Part model, mm, in its own coordinate system. A direction names the side the tool comes from. Coordinates: 2 decimals unless noted, no trailing zeros. Loops run counter-clockwise (first coordinate to the right, second up) from the corner with the lowest first, then second, coordinate; pieces in that order, holes last. Notation, with made-up numbers: M -23,6 L 16,6 A18 ccw 16,29 Z; hole C 28,46.25 d7. An arc over 180 degrees is marked long. Answer as CSV lines item,"result". Start each with the question number.
Autodesk Inventor part; units mm, degrees
ref_plane "Work Plane3" through (64.8592, 82.2824, 5) normal (0.5, 0, -0.866) x (0, 1, 0)
ref_plane "YZ Plane" through (0, 0, 0) normal (1, 0, 0) x (0, 1, 0)
ref_plane "XZ Plane" through (0, 0, 0) normal (0, 1, 0) x (-1, 0, 0)
sketch "Sketch1" plane through (0, 0, 0) normal (0, 0, 1) x (1, 0, 0)
  line L0 (0, 0) -> (55, 95.2628)
  line L1 (0, 0) -> (8.6603, 0)
  line L2 (64.8592, 0) -> (64.8592, 115) construction
  line L3 (64.8592, 0) -> (179.8592, 0) construction
  line L4 (56.1603, 82.2724) -> (65.4694, 82.2724) construction
  line L5 (79.2606, 82.2724) -> (79.2606, 95.2628)
  line L6 (55, 95.2628) -> (79.2606, 95.2628)
  line L7 (64.8592, 82.2724) -> (64.8592, 82.2824) construction
  line L8 (64.8592, 82.2824) -> (64.865, 82.2724)
  line L9 (64.8592, 82.2824) -> (64.8707, 82.2824) construction
  line L10 (64.8592, 82.2824) -> (64.8534, 82.2724)
  line L11 (64.8592, 82.2824) -> (64.8707, 82.2824) construction
  line L12 (64.865, 82.2724) -> (79.2606, 82.2724)
  line L13 (56.1603, 82.2724) -> (64.8534, 82.2724)
  line L14 (8.6603, 0) -> (53.6603, 0) construction
  line L15 (53.6603, 0) -> (32.0862, 40.5749)
  line L16 (53.6603, 0) -> (99.6142, 0) construction
  line L17 (36.5081, 48.2339) -> (62.1545, 0)
  line L18 (8.6603, 0) -> (32.0862, 40.5749)
  line L19 (36.5081, 48.2339) -> (56.1603, 82.2724)
  line L20 (62.1545, 0) -> (53.6603, 0)
  line L21 (79.2606, 95.2628) -> (79.2606, 82.2724) construction
  line L22 (64.8534, 82.2724) -> (64.865, 82.2724)
  dimension "d7" = 110
  dimension "d10" = 64.8592
  dimension "d11" = 115
  dimension "d12" = 90
  dimension "d15" = 95
  dimension "d22" = 0.01
  dimension "d23" = 60
  dimension "d24" = 120
  dimension "d27" = 45
  dimension "d28" = 118
  dimension "d29" = 7.5
  dimension "d43" = 7.5
  dimension "d44" = 7.5
  dimension "d45" = 24.2606
  dimension "d46" = 60
extrude "Extrusion2" add sketch "Sketch1" along normal blind 5 contours L0 L6 L5 L12 L8 L10 L13 L19 L17 L20 L15 L18 L1
ref_plane "Work Plane2" through (64.8592, 82.2824, 5) normal (0.866, 0, 0.5) x (0, 1, 0)
ref_plane "Work Plane1" through (79.2606, 95.2628, 5) normal (0.866, 0, 0.5) x (0, 1, 0)
sketch "Sketch2" plane through (64.8592, 82.2824, 5) normal (0.866, 0, 0.5) x (0, 1, 0)
  line L0 (12.9804, -7.2007) -> (12.9804, 4.9296) construction
  line L1 (-0.01, 0.0029) -> (0, 0) construction
  line L2 (0, 0) -> (12.9804, 0) construction
  circle A0 centre (12.9804, 0) radius 2
  point P0 (-82.2824, 28.0995)
  dimension "d33" = 4
ref_plane "Work Plane3" through (64.8592, 82.2824, 5) normal (0.5, 0, -0.866) x (0, 1, 0)
sketch "Sketch3" plane through (64.8592, 82.2824, 5) normal (0.5, 0, -0.866) x (0, 1, 0)
  line L0 (-101.735, 0) -> (34.4329, 0) construction
  line L1 (12.9804, -11.0383) -> (12.9804, 9.972) construction
  line L2 (12.9804, 12.472) -> (12.9804, -8.5383)
  line L3 (12.9804, 0) -> (12.9804, 3)
  line L4 (12.9804, 3) -> (7.7842, 0)
  line L5 (7.7842, 0) -> (12.9804, -3)
  line L6 (12.9804, -3) -> (12.9804, 3)
  point P0 (-82.2824, -58.6697)
  dimension "d38" = 3
  dimension "d39" = 60
  dimension "d40" = 60
extrude "Extrusion4" cut sketch "Sketch3" along normal through all both and the other way through all
sketch "Sketch4" plane through (79.2606, 95.2628, 5) normal (0, 1, 0) x (1, 0, 0)
  line L0 (-14.3957, 0) -> (0, 0) construction
  line L1 (0, 5) -> (-14.3957, 5) construction
  line L2 (-14.3957, 0) -> (-14.3957, 5) construction
  line L3 (-14.4072, 5) -> (-14.4072, 0) construction
  line L4 (-14.4072, 2.5) -> (-9.494, 2.5) construction
  line L5 (-8.0506, 5) -> (-10.9373, 0) construction
  line L6 (-11.5147, 5) -> (-14.4014, 0)
  circle A0 centre (-12.9581, 2.5) radius 1.25
  point P0 (-79.2606, 5)
  dimension "d47" = 2.5
extrude "Extrusion5" cut sketch "Sketch4" against normal through all
equation "\"d15\" = d7 - 2 * d9"
equation "\"d44\" = d43"
properties part number "TableSupport"
Q1. Slice it at D-D, the plane y = 57.5. Write the cut outline in (x, z).
Q2. Two-plate mould, pull along X, no slides. Class faces 6 (the face through (59, 95.263, 2)), 7 (the face through (27.115, 46.965, 2.465)), 8 (the face through (66.03, 87.33, 3.72)), 9 (the face through (64.27, 93.21, 2.39)): +X half, -X half, draft (parallel to the pull), parting line (faces both ways), or undercut.
Q3. Slice it at B-B, the plane x = 49.5. Write the cut outline in (y, z), and give its area (3 significant figures).
Q4. Slice it at A-A, the plane y = 22.5. Write the cut outline in (x, z), and give its area (3 significant figures).
Q5. Wall check: L1, parallel to Y at x = 39, z = 2.7; L2, parallel to Y at x = 56, z = 3.45; L3, parallel to X at y = 15, z = 3.75. Give the ranges that are in metal, low to high.
Q6. Tool access for faces 1 (the face through (20.209, 20.003, 2.465)), 2 (the face through (46.197, 65.015, 2.465)), 3 (the face through (79.261, 89, 2)), 4 (the face through (72, 82.272, 2)), 5 (the face through (58, 0, 2)): list every direction of +Z, -Z, +X, -X, +Y, -Y with a clear straight run to the whole face (end or side of a thin tool).
Q7. Flat gauge pins, fed straight in: P1, Ø1.5, axis at x = 30, z = 2, coming from the +Y side; P2, Ø1, axis at y = 15, z = 2, coming from the +X side; P3, Ø2.5, axis at x = 75.5, z = 2, coming from the -Y side. Where does each tip first touch, or does it go through?
Solved:
1,outline,"M 33.2,0 L 41.86,0 L 41.86,5 L 33.2,5 Z"
2,face 6,"draft"
2,face 7,"-X half"
2,face 8,"undercut"
2,face 9,"undercut"
3,outline,"M 7.82,0 L 23.8,0 L 23.8,5 L 7.82,5 Z; M 70.74,0 L 85.74,0 L 85.74,5 L 70.74,5 Z"
3,area,"155 mm2"
4,outline,"M 12.99,0 L 21.65,0 L 21.65,5 L 12.99,5 Z; M 41.7,0 L 50.19,0 L 50.19,5 L 41.7,5 Z"
4,area,"85.8 mm2"
5,L1,"y = 27.57 to 43.55, 52.55 to 67.55"
5,L2,"y = 0 to 11.57, 81.99 to 95.26"
5,L3,"x = 8.66 to 17.32, 45.68 to 54.18"
6,face 1,"+Z, -Z, -Y"
6,face 2,"+Z, -Z, +X"
6,face 3,"+Z, -Z, +X, +Y, -Y"
6,face 4,"+Z, -Z, +X, -Y"
6,face 5,"+Z, -Z, +X, -X, -Y"
7,P1,"stops at y = 53.26"
7,P2,"stops at x = 54.44"
7,P3,"stops at y = 82.27"
